from build123d import *

# Parameters (mm, degrees)
SKETCH1_R           = 14
BOSS_EXTRUDE1_DEPTH = 4
SKETCH2_R           = 2.975
CUT_EXTRUDE1_DEPTH  = 2
SKETCH3_R           = 11
CUT_EXTRUDE2_DEPTH  = 1
FILLET1_R           = 0.5
FILLET2_R           = 1.5


with BuildPart() as part:
    # Sketch1 → Boss-Extrude1 (new body)
    with BuildSketch(Plane.XY):
        Circle(SKETCH1_R)
    extrude(amount=BOSS_EXTRUDE1_DEPTH)

    # Sketch2 → Cut-Extrude1 (cut)
    with BuildSketch(Plane.XY.offset(4)):
        Circle(SKETCH2_R)
    extrude(amount=-CUT_EXTRUDE1_DEPTH, mode=Mode.SUBTRACT)

    # Sketch3 → Cut-Extrude2 (cut)
    with BuildSketch(Plane(origin=(0, 0, 0), x_dir=(-1, 0, 0), z_dir=(0, 0, -1))):
        Circle(SKETCH3_R)
    extrude(amount=-CUT_EXTRUDE2_DEPTH, mode=Mode.SUBTRACT)

    # Fillet1
    fillet1_edges = [part.edges().sort_by_distance(p)[0] for p in [
        (11, 0, 1),
        (11, 0, 0),
    ]]
    fillet(fillet1_edges, radius=FILLET1_R - 0.0001)  # a hair under: the kernel refuses the full size

    # Fillet2
    fillet2_edges = [part.edges().sort_by_distance(p)[0] for p in [
        (-14, 0, 0),
    ]]
    fillet(fillet2_edges, radius=FILLET2_R)


solid = part.part
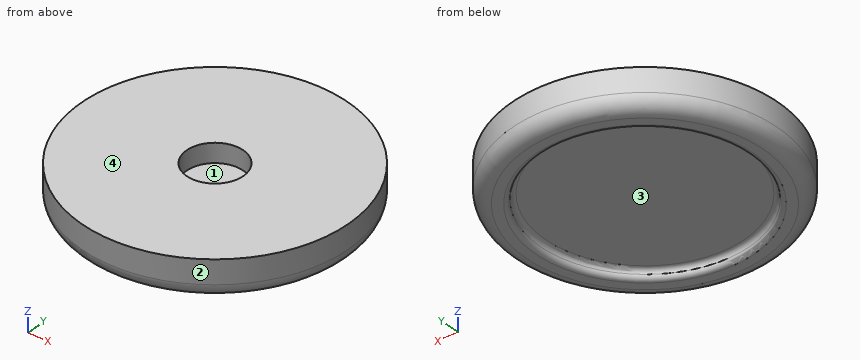
Input: part model. Units: mm. Frame: model coordinates. Face numbers are marked on the shaded views. Round coordinates to 2 decimals unless told otherwise and drop trailing zeros. Order: outer loops, then holes, each group sorted by start corner. A loop starts at its lowest first (then second) coordinate and runs counter-clockwise, first axis right, second up. Notation, with made-up numbers: (63, -16.75) - (101, -16.75) arc R5 cw to (101, -8.75) - close; hole circle Ø10 at (-32, 59). An arc over 180 degrees is marked (long way). Use a Markdown table: item, result.
1. Material intervals for probe 1 along Z at (x, y) = (1.5, -8); probe 2 along X at (y, z) = (-1.5, 3.4); probe 3 along X at (y, z) = (10, 0.6), sorted ascending.
Evaluation:
| item | result |
|---|---|
| probe 1 | 1 to 4 |
| probe 2 | -13.92 to -2.57, 2.57 to 13.92 |
| probe 3 | -9.36 to -4.56, 4.56 to 9.36 |
2. Mould query, pull axis X, two halves, no side actions, for the marked faces 1, 2, 3 and 4. Classes: +X half, -X half, draft (parallel to the pull), parting line (faces both ways), or undercut.
Evaluation:
| item | result |
|---|---|
| face 1 | undercut |
| face 2 | parting line |
| face 3 | undercut |
| face 4 | draft |
3. Section C-C on z = 3.25. Return the cut outline in (x, y) (3 decimals), then the cut area to 3 significant figures.
Evaluation:
| item | result |
|---|---|
| outline | circle Ø28 at (0, 0); hole circle Ø5.95 at (0, 0) |
| area | 588 mm^2 |
4. First-contact query: pin 1 (1.5 mm diameter, centred on x = 1.5, y = -2.5, fed in from -Z); pin 2 (7.5 mm diameter, centred on x = 0, y = 0, fed in from +Z); pin 3 (1.5 mm diameter, centred on x = -6.5, z = 3, fed in from +Y); pin 4 (2 mm diameter, centred on y = 5.5, z = 2.5, fed in from -X). Flat tips, straight axial feed; report the tip coordinate or a pass-through.
Evaluation:
| item | result |
|---|---|
| pin 1 | z = 1 |
| pin 2 | z = 4 |
| pin 3 | y = 12.76 |
| pin 4 | x = -13.26 |
